Autodesk Inventor part; units mm, degrees
ref_plane "YZ Plane" through (0, 0, 0) normal (1, 0, 0) x (0, 1, 0)
ref_plane "XZ Plane" through (0, 0, 0) normal (0, 1, 0) x (-1, 0, 0)
ref_plane "XY Plane" through (0, 0, 0) normal (0, 0, 1) x (1, 0, 0)
sketch "スケッチ1" plane through (0, 0, 0) normal (0, 1, 0) x (-1, 0, 0)
  line L0 (0, 0) -> (-45, 0)
  line L1 (-45, 0) -> (-45, 2)
  line L2 (-45, 2) -> (0, 2)
  line L3 (0, 2) -> (0, 0)
  dimension "d0" = 45
  dimension "d1" = 2
extrude "押し出し1" add sketch "スケッチ1" along normal blind 38
sketch "スケッチ2" plane through (0, 0, 2) normal (0, 0, 1) x (1, 0, 0)
  line L0 (45, 0) -> (0, 0)
  line L1 (45, 0) -> (45, 38)
  line L2 (0, 38) -> (45, 38)
  line L3 (45, 38) -> (45, 35)
  line L4 (45, 35) -> (0, 35)
  line L5 (0, 35) -> (0, 38)
  line L6 (0, 0) -> (45, 0)
  line L7 (45, 0) -> (45, 3)
  line L8 (45, 3) -> (0, 3)
  line L9 (0, 3) -> (0, 0)
  dimension "d4" = 3
  dimension "d5" = 3
extrude "押し出し2" add sketch "スケッチ2" along normal blind 50
sketch "スケッチ3" plane through (0, 38, 0) normal (0, 1, 0) x (1, 0, 0)
  line L0 (45, 0) -> (0, 0)
  line L1 (0, 0) -> (0, -52)
  line L2 (45, -52) -> (0, -52)
  line L3 (45, 0) -> (45, -52)
sketch "スケッチ4" plane through (0, 0, 0) normal (0, -1, 0) x (1, 0, 0)
  line L0 (0, 0) -> (45, 0)
  line L1 (14.737, 0) -> (29.997, 0)
  line L2 (29.997, 0) -> (29.997, 25.5)
  line L3 (29.997, 25.5) -> (14.737, 25.5)
  line L4 (14.737, 25.5) -> (14.737, 0)
  dimension "d8" = 15.26
  dimension "d9" = 25.5
hole "穴1" at (14.737, 0, 25.5) at (29.997, 0, 25.5) direction (0, 1, 0) diameter 3 depth 40 tip angle 118
properties part number "知能ロボコンギアボックス１"
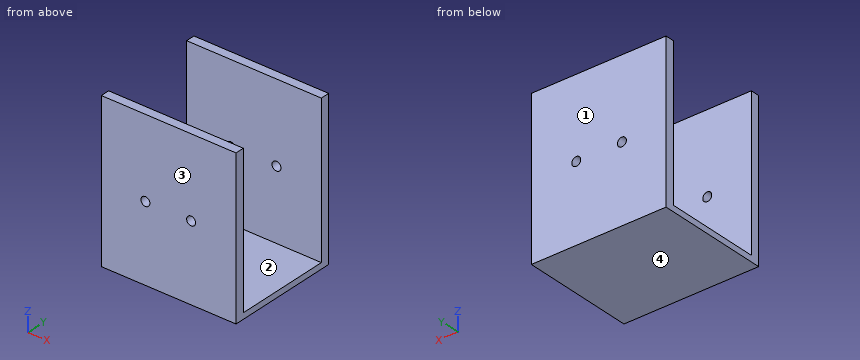
Input: part model. Units: mm. Frame: model coordinates. Face numbers are marked on the shaded views. Coordinates: 2 decimals unless noted, no trailing zeros. Loops run counter-clockwise (first coordinate to the right, second up) from the corner with the lowest first, then second, coordinate; pieces in that order, holes last. Notation, with made-up numbers: M 1.5,15 L 28.5,15 A23 cw 28.5,23 Z; hole C 33,-38.5 d5. An arc over 180 degrees is marked long. Answer in a Markdown table with one row per item.
1. Section C-C, the plane z = 8. Output: boundary loops of the cut face in (x, y), then the cut area to 3 significant figures.
Response:
| item | result |
|---|---|
| outline | M 0,0 L 45,0 L 45,3 L 0,3 Z; M 0,35 L 45,35 L 45,38 L 0,38 Z |
| area | 270 mm2 |
2. Section A-A, the plane z = 25.5. Output: boundary loops of the cut face in (x, y), then the cut area to 3 significant figures.
Response:
| item | result |
|---|---|
| outline | M 0,0 L 13.24,0 L 13.24,3 L 0,3 Z; M 0,35 L 13.24,35 L 13.24,38 L 0,38 Z; M 16.24,0 L 28.5,0 L 28.5,3 L 16.24,3 Z; M 16.24,35 L 28.5,35 L 28.5,38 L 16.24,38 Z; M 31.5,0 L 45,0 L 45,3 L 31.5,3 Z; M 31.5,35 L 45,35 L 45,38 L 31.5,38 Z |
| area | 234 mm2 |
3. Material intervals for line 1 (X direction, y = 35.9, z = 25.5); line 2 (Y direction, x = 42.5, z = 5.5); line 3 (Z direction, x = 8.5, y = 12.5), sorted ascending.
Response:
| item | result |
|---|---|
| line 1 | x = 0 to 13.24, 16.24 to 28.5, 31.5 to 45 |
| line 2 | y = 0 to 3, 35 to 38 |
| line 3 | z = 0 to 2 |
4. Section B-B, the plane x = 21.5. Output: boundary loops of the cut face in (y, z), then the cut area to 3 significant figures.
Response:
| item | result |
|---|---|
| outline | M 0,0 L 38,0 L 38,52 L 35,52 L 35,2 L 3,2 L 3,52 L 0,52 Z |
| area | 376 mm2 |
5. Draft query along Y for the marked faces 1, 2, 3 and 4. Return one class per face: pulls with the +Y half, pulls with the -Y half, needs draft (parallel to the pull), parting line crosses it, or undercut.
Response:
| item | result |
|---|---|
| face 1 | pulls with the +Y half |
| face 2 | undercut |
| face 3 | pulls with the -Y half |
| face 4 | needs draft |
6. Section D-D, the plane x = 14. Output: boundary loops of the cut face in (y, z), then the cut area to 3 significant figures.
Response:
| item | result |
|---|---|
| outline | M 0,0 L 38,0 L 38,24.19 L 35,24.19 L 35,2 L 3,2 L 3,24.19 L 0,24.19 Z; M 0,26.81 L 3,26.81 L 3,52 L 0,52 Z; M 35,26.81 L 38,26.81 L 38,52 L 35,52 Z |
| area | 360 mm2 |
